Can you work these out from the model? Positions are in its coordinate system, mm. A direction names the side the tool comes from. Round coordinates to 2 decimals unless told otherwise and drop trailing zeros. Order: outer loops, then holes, each group sorted by start corner. A loop starts at its lowest first (then second) coordinate and runs counter-clockwise, first axis right, second up. Notation, with made-up numbers: (40, 74) -> (49, 74) arc R14 cw to (49, 94) -> close; hole circle Ø10 at (53, 47). An arc over 180 degrees is marked (long way). One line per item, written item: value.
```python
from build123d import *

# Parameters (mm, degrees)
SM_BASE_FLANGE_1_DEPTH             = 8
SM_EDGE_FLANGE_1_STRIP_W           = 48
SM_EDGE_FLANGE_1_STRIP_H           = 8
SM_EDGE_FLANGE_1_STRIP_CUT_DEPTH   = 2335
SM_EDGE_FLANGE_1_STRIP_2_W         = 48
SM_EDGE_FLANGE_1_STRIP_2_H         = 8
SM_EDGE_FLANGE_1_STRIP_CUT_2_DEPTH = 2305
SM_EDGE_FLANGE_1_RELIEF_W          = 52
SM_EDGE_FLANGE_1_RELIEF_H          = 4
SM_EDGE_FLANGE_1_RELIEF_CUT_DEPTH  = 8
SM_EDGE_FLANGE_1_DEPTH             = 2335
SM_EDGE_FLANGE_1_BEND_DEPTH        = 2305
CHAMFER_1_SIZE                     = 4
SKETCH_12_R                        = 45
CUT_EXTRUDE_1_DEPTH                = 2347.241675531


# Sheet-metal steps are written as plain solids
with BuildPart() as part:
    # Sketch 1 → 基体-法兰1 (new body)
    with BuildSketch(Plane(origin=(0, 0, 0), x_dir=(0, 0, -1), z_dir=(1, 0, 0))):
        Polygon((0, 0), (2335, 0), (2335, -215), (30, -215), (0, -185), align=None)
    extrude(amount=-SM_BASE_FLANGE_1_DEPTH)

    # 边线-法兰1 strip (across the edge) → 边线-法兰1 strip cut (cut)
    with BuildSketch(Plane(origin=(-8, 0, 0), x_dir=(0, -1, 0), z_dir=(0, 0, -1))):
        with Locations((-8, -4)):
            Rectangle(SM_EDGE_FLANGE_1_STRIP_W, SM_EDGE_FLANGE_1_STRIP_H)
    extrude(amount=SM_EDGE_FLANGE_1_STRIP_CUT_DEPTH, mode=Mode.SUBTRACT)

    # 边线-法兰1 strip 2 (across the edge) → 边线-法兰1 strip cut 2 (cut)
    with BuildSketch(Plane(origin=(-8, -215, -2335), x_dir=(0, 1, 0), z_dir=(0, 0, 1))):
        with Locations((-8, -4)):
            Rectangle(SM_EDGE_FLANGE_1_STRIP_2_W, SM_EDGE_FLANGE_1_STRIP_2_H)
    extrude(amount=SM_EDGE_FLANGE_1_STRIP_CUT_2_DEPTH, mode=Mode.SUBTRACT)

    # 边线-法兰1 relief (on the sheet) → 边线-法兰1 relief cut (cut)
    with BuildSketch(Plane(origin=(-8, -199, -2335), x_dir=(0, 1, 0), z_dir=(-1, 0, 0))):
        with Locations((-22, -2307)):
            Rectangle(SM_EDGE_FLANGE_1_RELIEF_W, SM_EDGE_FLANGE_1_RELIEF_H)
    extrude(amount=-SM_EDGE_FLANGE_1_RELIEF_CUT_DEPTH, mode=Mode.SUBTRACT)

    # 边线-法兰1 section (across the edge) → 边线-法兰1 (add)
    with BuildSketch(Plane(origin=(-8, 0, 0), x_dir=(0, -1, 0), z_dir=(0, 0, -1))):
        with BuildLine():
            Line((0, 8), (0, 72))
            Line((0, 72), (8, 72))
            Line((8, 72), (8, 8))
            ThreePointArc((8, 8), (10.343145751, 2.343145751), (16, 0))
            Line((16, 0), (16, -8))
            ThreePointArc((16, -8), (4.686291501, -3.313708499), (0, 8))
        make_face()
    extrude(amount=SM_EDGE_FLANGE_1_DEPTH)

    # 边线-法兰1 section 2 (across the edge) → 边线-法兰1 bend (add)
    with BuildSketch(Plane(origin=(-8, -215, -2335), x_dir=(0, 1, 0), z_dir=(0, 0, 1))):
        with BuildLine():
            Line((0, 8), (0, 72))
            Line((0, 72), (8, 72))
            Line((8, 72), (8, 8))
            ThreePointArc((8, 8), (10.343145751, 2.343145751), (16, 0))
            Line((16, 0), (16, -8))
            ThreePointArc((16, -8), (4.686291501, -3.313708499), (0, 8))
        make_face()
    extrude(amount=SM_EDGE_FLANGE_1_BEND_DEPTH)

    # 倒角1
    chamfer_1_edges = [part.edges().sort_by_distance(p)[0] for p in [
        (-80, 0, -1167.5),
        (-80, -215, -1182.5),
    ]]
    chamfer(chamfer_1_edges, length=CHAMFER_1_SIZE)

    # 草图12 → 切除-拉伸1 (cut, through all)
    with BuildSketch(Plane(origin=(0, 0, 0), x_dir=(0, 0, -1), z_dir=(1, 0, 0))):
        with Locations((620, -107.5)):
            Circle(SKETCH_12_R)
    extrude(amount=-CUT_EXTRUDE_1_DEPTH, mode=Mode.SUBTRACT)


solid = part.part
```
Q1. We'd pull the mould along Y, two halves only. Please class faces 1 (the face through (-48, -8, -1151)), 2 (the face through (-46, 0, -1151)), 3 (the face through (-46, -215, -1199)): released by +Y, released by -Y, zero draft, split by the parting line, or undercut.
Answers below:
face 1: undercut
face 2: released by +Y
face 3: released by -Y
Q2. Please list where these lines run through material, in increasing order: line 1 along Y through (x, z) = (-48.5, -1148); line 2 along Y through (x, z) = (-5.5, -620); line 3 along X through (y, z) = (-60.5, -1259.5).
Answers below:
line 1: -215 to -207, -8 to 0
line 2: -211.07 to -152.5, -62.5 to -3.93
line 3: -8 to 0
Q3. I want a section at B-B on y = -107.5. List the corners of the cut face in (x, z) for me.
Answers below:
outline: (-8, -2335) -> (0, -2335) -> (0, -665) -> (-8, -665) -> close; (-8, -575) -> (0, -575) -> (0, 0) -> (-8, 0) -> close
Q4. Will these pins go through, and if not, where does the flat tip stop? pin 1 Ø8 at (y, z) = (-126, -2033.5) entering from -X; pin 2 Ø3 at (y, z) = (-36, -1424.5) entering from +X; pin 3 Ø22 at (x, y) = (-38.5, -203) entering from +Z.
Answers below:
pin 1: x = -8
pin 2: x = 0
pin 3: z = -30
Q5. I want a section at D-D on z = -2110.5. List the corners of the cut face in (x, y) for me, plus the area to 3 significant figures.
Answers below:
outline: (-80, -211) -> (-76, -215) -> (-16, -215) arc R16 ccw to (0, -199) -> (0, -16) arc R16 ccw to (-16, 0) -> (-76, 0) -> (-80, -4) -> (-80, -8) -> (-16, -8) arc R8 cw to (-8, -16) -> (-8, -199) arc R8 cw to (-16, -207) -> (-80, -207) -> close
area: 2,770 mm^2
Q6. On a 3-axis mill with a long thin cutter (end or side, diameter ignored), from which of +Z, -Z, +X, -X, +Y, -Y can I reach the whole of each face in a straight line? I mean faces 4 (the face through (-7.6, -115, -2335)), 5 (the face through (-8, -112, -1184)). Say none if no direction works.
Answers below:
face 4: -Z, +X, -X, +Y, -Y
face 5: +Z, -Z, -X
Q7. I want a section at C-C on x = -30.5. List the corners of the cut face in (y, z) for me, plus the area to 3 significant figures.
Answers below:
outline: (-215, -2335) -> (-207, -2335) -> (-207, -30) -> (-215, -30) -> close; (-8, -2335) -> (0, -2335) -> (0, 0) -> (-8, 0) -> close
area: 37,100 mm^2
Q8. I want a section at A-A on z = -620. List the corners of the cut face in (x, y) for me.
Answers below:
outline: (-80, -211) -> (-76, -215) -> (-16, -215) arc R16 ccw to (0, -199) -> (0, -152.5) -> (-8, -152.5) -> (-8, -199) arc R8 cw to (-16, -207) -> (-80, -207) -> close; (-80, -8) -> (-16, -8) arc R8 cw to (-8, -16) -> (-8, -62.5) -> (0, -62.5) -> (0, -16) arc R16 ccw to (-16, 0) -> (-76, 0) -> (-80, -4) -> close
